Could you check a few things on this drawing? It's one solid part, dimensions in mm from its lowest x, y, z. A direction names the side the tool comes from. Coordinates: 2 decimals unless noted, no trailing zeros. Order: outer loops, then holes, each group sorted by start corner. A loop starts at its lowest first (then second) coordinate and runs counter-clockwise, first axis right, second up. Notation, with made-up numbers: (59.5, 82.5) -> (105.5, 82.5) arc R17 cw to (105.5, 107.5) -> close; hole circle Ø6 at (-0.75, -15). An arc over 180 degrees is marked (long way). Use a Markdown table: item, result. Add a question column.
1. For the marked faces 1 and 2, which set-ups out of +Z, -Z, +X, -X, +Y, -Y let a thin tool reach every point of the face, with its end or its side?
2. If I drill on line 1 along X through (y, z) = (135.5, 43.5); line 2 along Y through (x, z) = (58.5, 69); line 3 along Y through (x, z) = (7, 18), over which ranges is the centre line in solid material (lowest first)? Write a range as from..to.
3. Suppose I cut it at C-C, the plane z = 13.5. List the corners of the cut face in (x, y) for me, then the cut area to 3 significant figures.
4. Suppose I cut it at D-D, the plane x = 112.5. List the corners of the cut face in (y, z) for me, then the cut area to 3 significant figures.
5. We'd pull the mould along Y, two halves only. Please class the marked faces 3, 4 and 5: pulls with the +Y half, pulls with the -Y half, needs draft (parallel to the pull), parting line crosses it, or undercut.
6. Suppose I cut it at B-B, the plane y = 117. List the corners of the cut face in (x, z) for me.
7. Suppose I cut it at A-A, the plane x = 60. List the corners of the cut face in (y, z) for me.
8. For pin 1 Ø6 at (x, z) = (12, 55.5) entering from +Y; pin 2 Ø6 at (x, z) = (14.5, 45.5) entering from -Y; pin 3 Ø10 at (x, y) = (68, 141.5) entering from +Z; pin 4 Ø11 at (y, z) = (55.5, 33.5) entering from +X, each with a flat end and sliding along its axis, tell me the tip position at first contact or that it passes through.
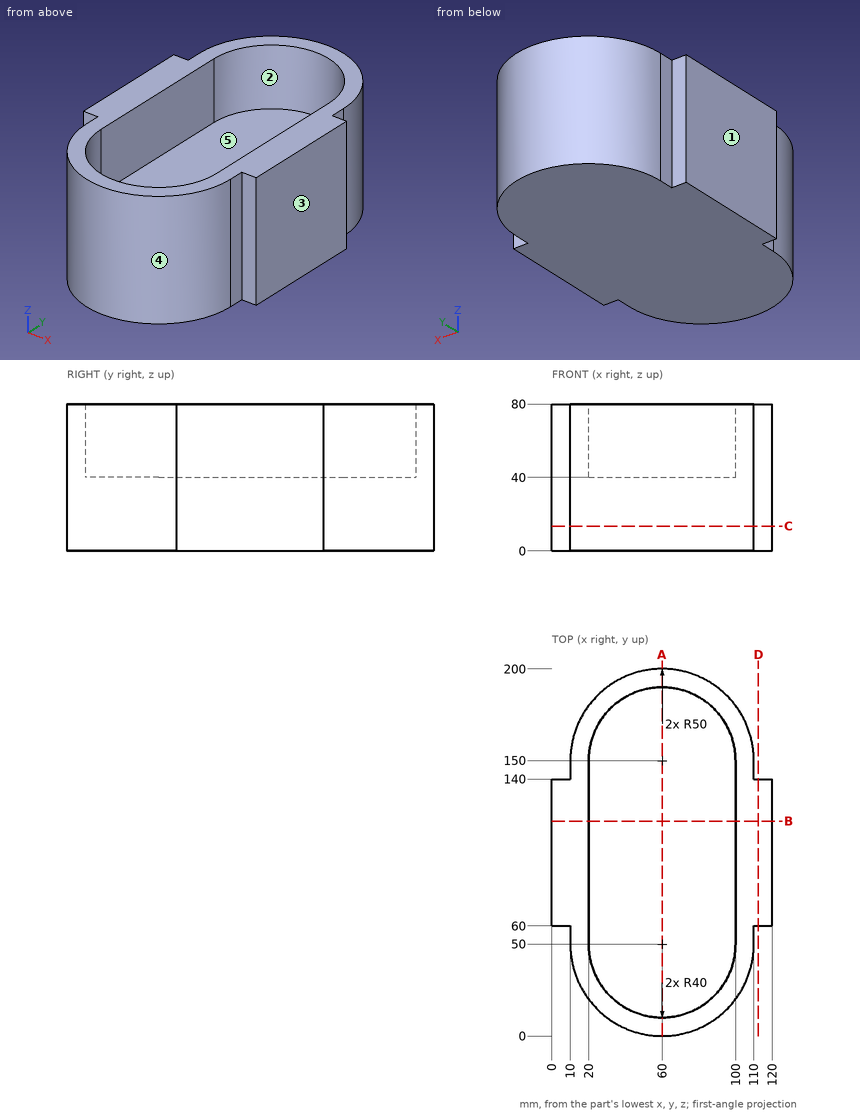
Worked out:
| question | item | result |
|---|---|---|
| 1 | face 1 | +Z, -Z, -X, +Y, -Y |
| 1 | face 2 | +Z |
| 2 | line 1 | x = 0..20, 100..120 |
| 2 | line 2 | y = 0.02..10.03, 189.97..199.98 |
| 2 | line 3 | y = 60..140 |
| 3 | outline | (0, 60) -> (10, 60) -> (10, 50) arc R50 ccw to (110, 50) -> (110, 60) -> (120, 60) -> (120, 140) -> (110, 140) -> (110, 150) arc R50 ccw to (10, 150) -> (10, 140) -> (0, 140) -> close |
| 3 | area | 19,500 mm² |
| 4 | outline | (60, 0) -> (140, 0) -> (140, 80) -> (60, 80) -> close |
| 4 | area | 6,400 mm² |
| 5 | face 3 | needs draft |
| 5 | face 4 | pulls with the -Y half |
| 5 | face 5 | undercut |
| 6 | outline | (0, 0) -> (120, 0) -> (120, 80) -> (100, 80) -> (100, 40) -> (20, 40) -> (20, 80) -> (0, 80) -> close |
| 7 | outline | (0, 0) -> (200, 0) -> (200, 80) -> (190, 80) -> (190, 40) -> (10, 40) -> (10, 80) -> (0, 80) -> close |
| 8 | pin 1 | stops at y = 171.79 |
| 8 | pin 2 | stops at y = 23.66 |
| 8 | pin 3 | stops at z = 40 |
| 8 | pin 4 | stops at x = 120 |
